from build123d import *

# Parameters (mm, degrees)
SKETCH1_R               = 44.45
SKETCH1_R_2             = 42.45
BOSS_EXTRUDE1_DEPTH     = 37.5
CUT_EXTRUDE1_REACH      = 75.197
CUT_EXTRUDE1_END_RADIUS = 44.45
SKETCH2_W               = 8
SKETCH2_H               = 16
SKETCH3_R               = 4
CUT_EXTRUDE2_DEPTH      = 74.197370171


with BuildPart() as part:
    # Sketch1 → Boss-Extrude1 (new, symmetric)
    with BuildSketch(Plane(origin=(0, 0, 0), x_dir=(1, 0, 0), z_dir=(0, 1, 0))):
        with Locations(Location((0, 0, 0), (0, 0, 270))):
            Circle(SKETCH1_R)
        with Locations(Location((0, 0, 0), (0, 0, 270))):
            Circle(SKETCH1_R_2, mode=Mode.SUBTRACT)
    extrude(amount=BOSS_EXTRUDE1_DEPTH, both=True)

    # Cut-Extrude1: up to this cylinder (the profile starts inside it)
    cut_extrude1_end = Plane(origin=(0, -37.5, 0), z_dir=(0, -1, 0)) * Cylinder(CUT_EXTRUDE1_END_RADIUS, 240.294, mode=Mode.PRIVATE)
    # Sketch2 → Cut-Extrude1 (cut, up to the surface)
    with BuildSketch(Plane(origin=(0, 0, 0), x_dir=(0, 0, -1), z_dir=(1, 0, 0)), mode=Mode.PRIVATE) as cut_extrude1_sk1:
        with Locations((0, -37.5)):
            Rectangle(SKETCH2_W, SKETCH2_H)
    cut_extrude1_tool1 = extrude(cut_extrude1_sk1.sketch, amount=-CUT_EXTRUDE1_REACH, mode=Mode.PRIVATE) & cut_extrude1_end
    add(cut_extrude1_tool1.solids().sort_by_distance((0, -37.5, 0))[0], mode=Mode.SUBTRACT)

    # Sketch3 → Cut-Extrude2 (cut, through all)
    with BuildSketch(Plane(origin=(0, 0, 0), x_dir=(0, 0, -1), z_dir=(1, 0, 0))):
        with Locations(Location((0, -20.55, 0), (0, 0, 180))):
            Circle(SKETCH3_R)
    extrude(amount=CUT_EXTRUDE2_DEPTH, mode=Mode.SUBTRACT)


solid = part.part
The model under review builds one solid part; all positions refer to its coordinate system, in mm. A direction names the side the tool comes from. Give positions to 0.01 mm unless a question says otherwise; leave off trailing zeros. Order: outer loops, then holes, each group sorted by start corner. A loop starts at its lowest first (then second) coordinate and runs counter-clockwise, first axis right, second up. Notation, with made-up numbers: (-8.5, -26.75) -> (47.5, -26.75) arc R29 cw to (47.5, 2.25) -> close; hole circle Ø11 at (24.5, -34.75). An arc over 180 degrees is marked (long way). Write item = value, one per line. Start each with the question number.
(1) For pin 1 Ø3 at (y, z) = (-13.5, -18.5) entering from +X; pin 2 Ø10.5 at (y, z) = (-20.55, 0) entering from -X; pin 3 Ø5 at (x, y) = (-25, 4) entering from +Z, all flat-tipped, find the tip position at first contact; note any pin that passes through.
(2) Tool access review of faces 4 (the flat face through (0, -37.5, 43)), 5 (the cylindrical face through (43.34, -20.726, -3.996)): name each direction out of +Z, -Z, +X, -X, +Y, -Y from which nothing blocks a thin tool from reaching the whole face with its end or side.
(3) Take a section at B-B (x = 0). Write out the cut boundary in (y, z), plus the area to 3 significant figures.
(4) Take a section at D-D (z = 16). Write out the cut boundary in (x, y), plus the area to 3 significant figures.
(5) Draft analysis for pull direction Z (two halves, no side actions). For faces 1 (the cylindrical face through (37.48, 0.52, 23.9)), 2 (the flat face through (-36, 37.5, 23)), 3 (the cylindrical face through (42.09, -0.52, -5.53)), state which applies: +Z half, -Z half, draft (parallel to the pull), parting line (faces both ways), or undercut.
(6) Take a section at A-A (z = 0). Write out the cut boundary in (x, y), plus the area to 3 significant figures.
(7) Take a section at C-C (y = -10.5). Write out the cut boundary in (x, z), plus the area to 3 significant figures.
(8) For L1, parallel to Y at x = 43, z = 0; L2, parallel to X at y = -16, z = 0; L3, parallel to Z at x = -38.5, y = 18, list the stretches that pass through material, from the lowest coordinate up. Write a range as from..to.
Returned:
q1.pin_1 = 41.07
q1.pin_2 = -44.45
q1.pin_3 = 38.33
q2.face_4 = +Z, -Z, +X, -X, -Y
q2.face_5 = +X
q3.outline = (-37.5, -44.45) -> (37.5, -44.45) -> (37.5, -42.45) -> (-37.5, -42.45) -> close; (-37.5, 42.45) -> (37.5, 42.45) -> (37.5, 44.45) -> (-37.5, 44.45) -> close
q3.area = 300 mm²
q4.outline = (-41.47, -37.5) -> (-39.32, -37.5) -> (-39.32, 37.5) -> (-41.47, 37.5) -> close; (39.32, -37.5) -> (41.47, -37.5) -> (41.47, 37.5) -> (39.32, 37.5) -> close
q4.area = 323 mm²
q5.face_1 = parting line
q5.face_2 = draft
q5.face_3 = undercut
q6.outline = (-44.45, -29.5) -> (-42.45, -29.5) -> (-42.45, 37.5) -> (-44.45, 37.5) -> close; (42.45, -37.5) -> (44.45, -37.5) -> (44.45, -24.55) -> (42.45, -24.55) -> close; (42.45, -16.55) -> (44.45, -16.55) -> (44.45, 37.5) -> (42.45, 37.5) -> close
q6.area = 268 mm²
q7.outline = circle Ø88.9 at (0, 0); hole circle Ø84.9 at (0, 0)
q7.area = 546 mm²
q8.L1 = -37.5..-24.55, -16.55..37.5
q8.L2 = -44.45..-42.45, 42.45..44.45
q8.L3 = -22.22..-17.88, 17.88..22.22
